Design review of the part built by this model. Coordinates are the model's own, in mm. Face numbers are marked on the shaded views. A direction names the side the tool comes from. Round coordinates to 2 decimals unless told otherwise and drop trailing zeros. Order: outer loops, then holes, each group sorted by start corner. A loop starts at its lowest first (then second) coordinate and runs counter-clockwise, first axis right, second up. Notation, with made-up numbers: (0.5, 41.5) - (25.5, 41.5) arc R17 ccw to (25.5, 51.5) - close; hole circle Ø7 at (43, 41.5). An arc over 180 degrees is marked (long way). Write item = value, one per line.
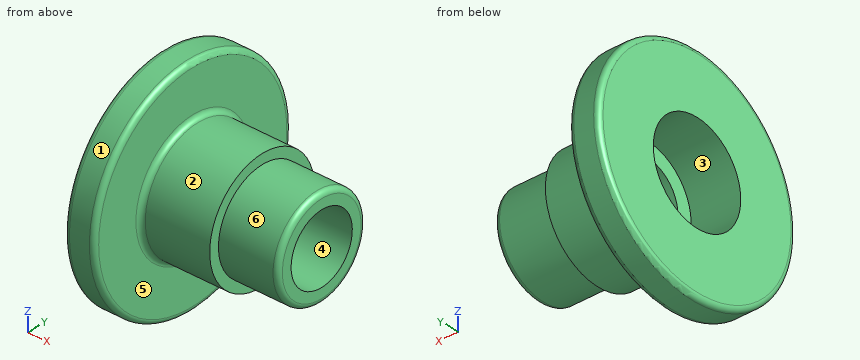
from build123d import *

# Parameters (mm, degrees)
FILLET1_R             = 0.5
M8X1_0_TAPPED_HOLE1_D = 7
SKETCH4_R             = 5
CUT_EXTRUDE1_DEPTH    = 5


with BuildPart() as part:
    # Sketch1 → Revolve1 (revolve)
    with BuildSketch(Plane.XY):
        Polygon((0, 0), (0, 11.25), (3, 11.25), (3, 6), (10, 6), (10, 5), (16, 5), (16, 0), align=None)
    revolve(axis=Axis((0, 0, 0), (1, 0, 0)))

    # Fillet1
    fillet1_edges = [part.edges().sort_by_distance(p)[0] for p in [
        (16, -5, 0),
        (3, -6, 0),
        (3, -11.25, 0),
        (0, -11.25, 0),
    ]]
    fillet(fillet1_edges, radius=FILLET1_R)

    # M8x1.0 Tapped Hole1 (through all)
    with Locations(Plane(origin=(16, 0, 0), x_dir=(0, 0, -1), z_dir=(1, 0, 0))):
        with Locations((0, 0)):
            Hole(M8X1_0_TAPPED_HOLE1_D / 2)

    # Sketch4 → Cut-Extrude1 (cut)
    with BuildSketch(Plane.ZY):
        Circle(SKETCH4_R)
    extrude(amount=-CUT_EXTRUDE1_DEPTH, mode=Mode.SUBTRACT)


solid = part.part
1) Clearance check with flat-ended pins moving along their axes: pin 1 Ø2 at (x, z) = (14, -1) entering from +Y; pin 2 Ø1 at (y, z) = (5.5, 1) entering from +X; pin 3 Ø1.5 at (x, y) = (3, 4) entering from +Z. State where each tip first meets the part, or that it passes through.
Findings:
pin_1 = 5
pin_2 = 10
pin_3 = 10.72
2) The part is to be moulded in two halves that separate along Z. For the marked faces 4, 5 and 6, say which applies: released by +Z, released by -Z, zero draft, split by the parting line, or undercut.
Findings:
face_4 = undercut
face_5 = zero draft
face_6 = split by the parting line
3) We need section A-A on z = 0. Write out the cut boundary in (x, y), and give its area (3 significant figures).
Findings:
outline = (0, -10.75) arc R0.5 ccw to (0.5, -11.25) - (2.5, -11.25) arc R0.5 ccw to (3, -10.75) - (3, -6.5) arc R0.5 cw to (3.5, -6) - (10, -6) - (10, -5) - (15.5, -5) arc R0.5 ccw to (16, -4.5) - (16, -3.5) - (5, -3.5) - (5, -5) - (0, -5) - close; (0, 5) - (5, 5) - (5, 3.5) - (16, 3.5) - (16, 4.5) arc R0.5 ccw to (15.5, 5) - (10, 5) - (10, 6) - (3.5, 6) arc R0.5 cw to (3, 6.5) - (3, 10.75) arc R0.5 ccw to (2.5, 11.25) - (0.5, 11.25) arc R0.5 ccw to (0, 10.75) - close
area = 84.3 mm^2
4) We need section D-D on x = 13.5. Write out the cut boundary in (y, z), and give its area (3 significant figures).
Findings:
outline = circle Ø10 at (0, 0); hole circle Ø7 at (0, 0)
area = 40.1 mm^2
5) To check wall thickness, follow L1, parallel to Y at x = 2, z = 1.25; L2, parallel to X at y = 6, z = 8; L3, parallel to Z at x = 9, y = 1.25. State the ranges of each line that lie inside material, in increasing order. Write a range as from..to.
Findings:
L1 = -11.18..-4.84, 4.84..11.18
L2 = 0..3
L3 = -5.87..-3.27, 3.27..5.87
6) For the marked faces 1, 2 and 3, list the 3-axis set-ups (+Z, -Z, +X, -X, +Y, -Y) from which the entire face can be reached by the end or side of a thin tool; tool diameter is ignored.
Findings:
face_1 = +X, -X
face_2 = +X
face_3 = -X
7) We need section C-C on x = 4.5. Write out the cut boundary in (y, z), and give its area (3 significant figures).
Findings:
outline = circle Ø12 at (0, 0); hole circle Ø10 at (0, 0)
area = 34.6 mm^2
